Here's the drawing with two shaded views (mm, measured from the low corner). I have some questions. Round coordinates to 2 decimals unless told otherwise and drop trailing zeros. Write each loop counter-clockwise with the first axis right and the second up, starting at its lowest first coordinate (ties: lowest second). Pieces come first, ordered by that corner, then holes.
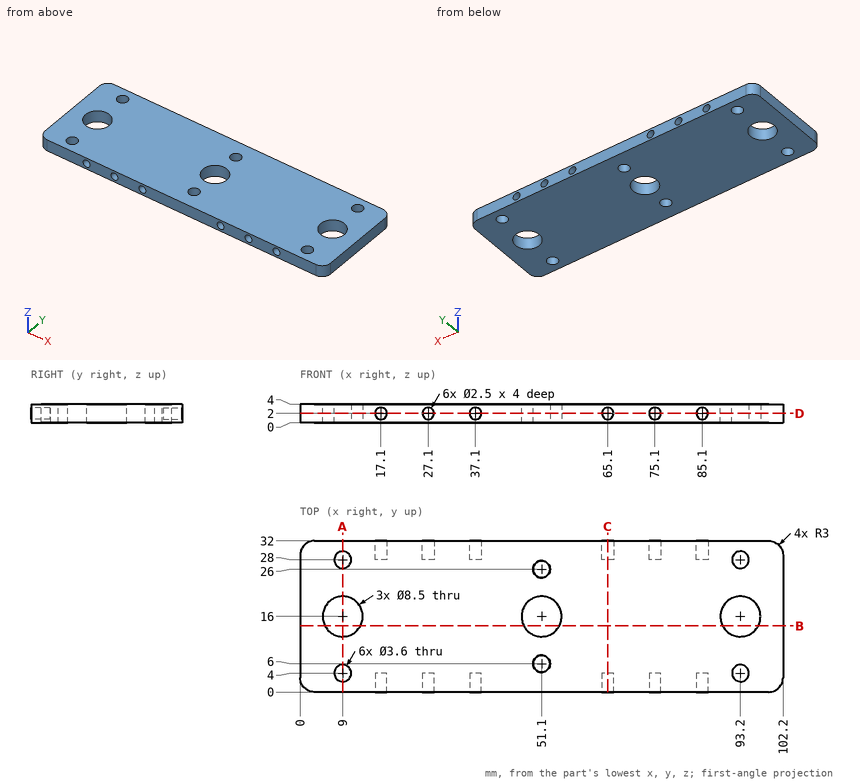
Q1. I'm going to push flat-ended pins straight in: pin 1 Ø2 at (x, y) = (9, 28) entering from +Z; pin 2 Ø2 at (x, z) = (65.5, 1.5) entering from +Y; pin 3 Ø2 at (x, z) = (27.1, 2) entering from +Y; pin 4 Ø2 at (x, z) = (65, 2) entering from -Y. Where does each tip first touch, or does it pass through?
Q2. If I drill on L1, parallel to Y at x = 51.1, z = 1.25; L2, parallel to Y at x = 93.2, z = 2.15; L3, parallel to X at y = 26, z = 1.4, over which ranges is the centre line in solid material (lowest first)?
Q3. Imagine slicing it at C-C, the plane x = 65.1. Write out the boundary of the cut face in (y, z).
Q4. Imagine slicing it at D-D, the plane z = 2. Count the separate pieces of the cut face and the enclosed holes in it, then the cut area to 3 significant figures.
Q5. Imagine slicing it at B-B, the plane y = 14. Write out the boundary of the cut face in (x, z), then the cut area to 3 significant figures.
Q6. Imagine slicing it at A-A, the plane x = 9. Write out the boundary of the cut face in (y, z).
Results found:
1. pin 1: passes through
1. pin 2: stops at y = 32
1. pin 3: stops at y = 28
1. pin 4: stops at y = 4
2. L1: y = 0 to 4.2, 7.8 to 11.75, 20.25 to 24.2, 27.8 to 32
2. L2: y = 0 to 2.2, 5.8 to 11.75, 20.25 to 26.2, 29.8 to 32
2. L3: x = 0 to 49.3, 52.9 to 102.2
3. outline: (0, 0) - (32, 0) - (32, 0.75) - (28, 0.75) - (28, 3.25) - (32, 3.25) - (32, 4) - (0, 4) - (0, 3.25) - (4, 3.25) - (4, 0.75) - (0, 0.75) - close
4. separate pieces: 1
4. enclosed holes: 9
4. area: 2,910 mm2
5. outline: (0, 0) - (5.25, 0) - (5.25, 4) - (0, 4) - close; (12.75, 0) - (47.35, 0) - (47.35, 4) - (12.75, 4) - close; (54.85, 0) - (89.45, 0) - (89.45, 4) - (54.85, 4) - close; (96.95, 0) - (102.2, 0) - (102.2, 4) - (96.95, 4) - close
5. area: 319 mm2
6. outline: (0, 0) - (2.2, 0) - (2.2, 4) - (0, 4) - close; (5.8, 0) - (11.75, 0) - (11.75, 4) - (5.8, 4) - close; (20.25, 0) - (26.2, 0) - (26.2, 4) - (20.25, 4) - close; (29.8, 0) - (32, 0) - (32, 4) - (29.8, 4) - close
